Source: three-view drawing plus pictorial views. Frame: mm from the lowest corner of the part. A direction names the side the tool comes from. Coordinates: 2 decimals unless noted, no trailing zeros. Order: outer loops, then holes, each group sorted by start corner. A loop starts at its lowest first (then second) coordinate and runs counter-clockwise, first axis right, second up. Notation, with made-up numbers: M -8.75,84 L 36.25,84 A27 cw 36.25,122 Z; hole C -3,22 d8. An arc over 180 degrees is marked long. One line per question, with ' | ' between items.
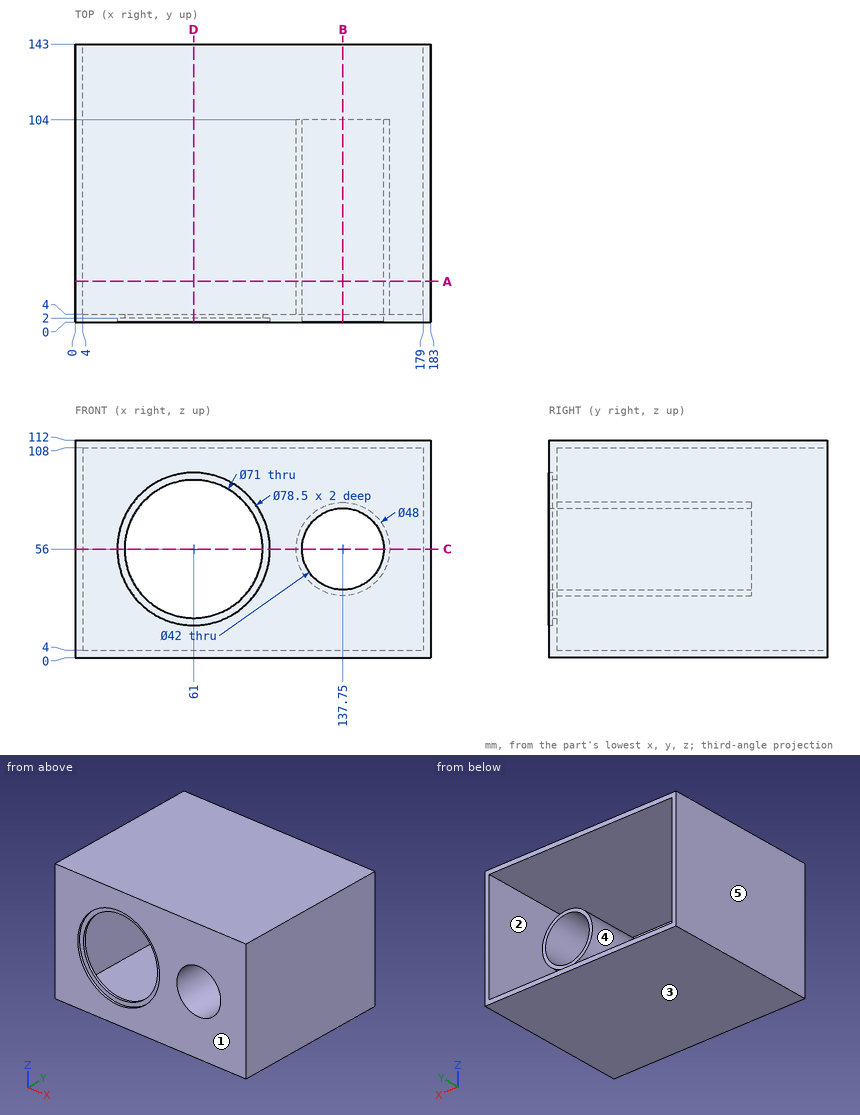
1. Draft query along Z for the marked faces 3, 4 and 5. Return one class per face: pulls with the +Z half, pulls with the -Z half, needs draft (parallel to the pull), parting line crosses it, or undercut.
Response values:
face 3: pulls with the -Z half | face 4: undercut | face 5: needs draft
2. Section D-D, the plane x = 61. Output: boundary loops of the cut face in (y, z), and give its area (3 significant figures).
Response values:
outline: M 0,0 L 143,0 L 143,4 L 4,4 L 4,20.5 L 2,20.5 L 2,16.75 L 0,16.75 Z; M 0,95.25 L 2,95.25 L 2,91.5 L 4,91.5 L 4,108 L 143,108 L 143,112 L 0,112 Z | area: 1,260 mm^2
3. Section C-C, the plane z = 56. Output: boundary loops of the cut face in (x, y), and give its area (3 significant figures).
Response values:
outline: M 0,0 L 21.75,0 L 21.75,2 L 25.5,2 L 25.5,4 L 4,4 L 4,143 L 0,143 Z; M 96.5,2 L 100.25,2 L 100.25,0 L 116.75,0 L 116.75,104 L 113.75,104 L 113.75,4 L 96.5,4 Z; M 158.75,0 L 183,0 L 183,143 L 179,143 L 179,4 L 161.75,4 L 161.75,104 L 158.75,104 Z | area: 1,980 mm^2
4. Section A-A, the plane y = 21. Output: boundary loops of the cut face in (x, z).
Response values:
outline: M 0,0 L 183,0 L 183,112 L 0,112 Z; C 137.75,56 d48; hole M 4,4 L 179,4 L 179,108 L 4,108 Z; hole C 137.75,56 d42
5. Pin query (flat end, axial travel): P1, Ø3, axis at x = 111, y = 75, coming from the -Z side; P2, Ø1, axis at x = 47.5, z = 87.5, coming from the -Y side; P3, Ø14.5, axis at x = 126, z = 47.5, coming from the +Y side. Return the tip coordinate at first contact, or that it passes through.
Response values:
P1: stops at z = 0 | P2: passes through | P3: stops at y = 104
6. Access query for the marked faces 1 and 2. Directions: +Z, -Z, +X, -X, +Y, -Y. A direction counts if a zero-diameter tool reaches every point of the face in a straight line with its end or side. Return the directions, or none.
Response values:
face 1: +Z, -Z, +X, -X, -Y | face 2: +Y
7. Material intervals for line 1 (X direction, y = 9, z = 56); line 2 (Z direction, x = 137, y = 76); line 3 (X direction, y = 1, z = 56), sorted ascending. Write a range as [from, to].
Response values:
line 1: x = [0, 4], [113.75, 116.75], [158.75, 161.75], [179, 183] | line 2: z = [0, 4], [32.01, 35.01], [76.99, 79.99], [108, 112] | line 3: x = [0, 21.75], [100.25, 116.75], [158.75, 183]
8. Section B-B, the plane x = 137.75. Output: boundary loops of the cut face in (y, z), and give its area (3 significant figures).
Response values:
outline: M 0,0 L 143,0 L 143,4 L 4,4 L 4,32 L 104,32 L 104,35 L 0,35 Z; M 0,77 L 104,77 L 104,80 L 4,80 L 4,108 L 143,108 L 143,112 L 0,112 Z | area: 1,990 mm^2
